```python
from build123d import *

# Parameters (mm, degrees)
F1_DEPTH     = 10
F2_DEPTH     = 8
F3_R         = 3
F4_T1_DEPTH  = 21.25
F4_T4_ANGLE  = 90
F4_T6_ANGLE  = 90
F4_T8_ANGLE  = 90
F4_T10_ANGLE = 90
F4_T12_ANGLE = 90
F4_T14_ANGLE = 90
F4_T16_ANGLE = 90
F4_T18_ANGLE = 90


# Not quite as in the source:
# - a fillet or chamfer that OpenCascade refuses, or shapes differently, is made with other operations: its cross-section is extruded or revolved along the edge and cut away or added


with BuildPart() as f1:
    # F0 (on Top) → F1 (new body)
    with BuildSketch(Plane.XY):
        Polygon((25.7107810123, -8.5209181738), (27.2851523571, -8.9427697042), (27.7070038876, -10.5171410491), (33.0728534806, -15.8829906421), (49.6898628385, 0.7340187158), (36.9619407771, 13.4619407771), (20.3449314192, -3.1550685808), align=None)
        Polygon((33.0728534806, -15.8829906421), (27.7070038876, -10.5171410491), (29.8254495283, -18.4232878133), (22.8852285904, -25.3635087511), (14.9790818262, -23.2450631104), (20.3449314192, -28.6109127035), align=None)
        Polygon((17.8046342481, -6.4024725331), (25.7107810123, -8.5209181738), (20.3449314192, -3.1550685808), (7.6170093579, -15.8829906421), (12.9828589509, -21.2488402351), (10.8644133102, -13.342693471), align=None)
        Polygon((49.6898628385, -32.5), (33.0728534806, -15.8829906421), (20.3449314192, -28.6109127035), (36.9619407771, -45.2279220614), align=None)
        Polygon((7.6170093579, -15.8829906421), (20.3449314192, -3.1550685808), (3.7279220614, 13.4619407771), (-9, 0.7340187158), align=None)
        Polygon((3.7279220614, -45.2279220614), (20.3449314192, -28.6109127035), (14.9790818262, -23.2450631104), (13.4047104814, -22.82321158), (12.9828589509, -21.2488402351), (7.6170093579, -15.8829906421), (-9, -32.5), align=None)
        Polygon((29.8254495283, -18.4232878133), (27.7070038876, -10.5171410491), (25.7107810123, -8.5209181738), (17.8046342481, -6.4024725331), (10.8644133102, -13.342693471), (12.9828589509, -21.2488402351), (14.9790818262, -23.2450631104), (22.8852285904, -25.3635087511), align=None)
        Polygon((27.7070038876, -10.5171410491), (27.2851523571, -8.9427697042), (25.7107810123, -8.5209181738), align=None)
        Polygon((13.4047104814, -22.82321158), (14.9790818262, -23.2450631104), (12.9828589509, -21.2488402351), align=None)
    extrude(amount=F1_DEPTH)

    # F0 (on Top) → F2 (cut)
    with BuildSketch(Plane.XY):
        Polygon((29.8254495283, -18.4232878133), (27.7070038876, -10.5171410491), (25.7107810123, -8.5209181738), (17.8046342481, -6.4024725331), (10.8644133102, -13.342693471), (12.9828589509, -21.2488402351), (14.9790818262, -23.2450631104), (22.8852285904, -25.3635087511), align=None)
        Polygon((13.4047104814, -22.82321158), (14.9790818262, -23.2450631104), (12.9828589509, -21.2488402351), align=None)
        Polygon((27.7070038876, -10.5171410491), (27.2851523571, -8.9427697042), (25.7107810123, -8.5209181738), align=None)
    extrude(amount=F2_DEPTH, mode=Mode.SUBTRACT)

    # F3
    f3_edges = [f1.edges().sort_by_distance(p)[0] for p in [
        (43.325902, 7.09798, 10),
        (28.653436, 5.153436, 10),
        (12.036427, 5.153436, 10),
        (-2.636039, 7.09798, 10),
        (-0.691495, -7.574486, 10),
        (-0.691495, -24.191495, 10),
        (-2.636039, -38.863961, 10),
        (12.036427, -36.919417, 10),
        (28.653436, -36.919417, 10),
        (43.325902, -38.863961, 10),
        (41.381358, -24.191495, 10),
        (41.381358, -7.574486, 10),
    ]]
    fillet(f3_edges, radius=F3_R)

    # F4: fillet of radius 4.5 on 8 edges, made by hand

    # F4_s2 → F4_t1 (cut)
    with BuildSketch(Plane.XY.offset(-11.25)):
        with BuildLine():
            ThreePointArc((40.1439212925, 10.2799602618), (36.9619407771, 11.5979797464), (33.7799602618, 10.2799602618))
            Line((33.7799602618, 10.2799602618), (36.9619407771, 13.4619407771))
            Line((36.9619407771, 13.4619407771), (40.1439212925, 10.2799602618))
        make_face()
        with BuildLine():
            ThreePointArc((46.5078823231, 3.9159992311), (47.8259018078, 0.7340187158), (46.5078823231, -2.4479617996))
            Line((46.5078823231, -2.4479617996), (49.6898628385, 0.7340187158))
            Line((49.6898628385, 0.7340187158), (46.5078823231, 3.9159992311))
        make_face()
        with BuildLine():
            ThreePointArc((46.5078823231, -29.3180194847), (47.8259018078, -32.5), (46.5078823231, -35.6819805153))
            Line((46.5078823231, -35.6819805153), (49.6898628385, -32.5))
            Line((49.6898628385, -32.5), (46.5078823231, -29.3180194847))
        make_face()
        with BuildLine():
            ThreePointArc((40.1439212925, -42.045941546), (36.9619407771, -43.3639610307), (33.7799602618, -42.045941546))
            Line((33.7799602618, -42.045941546), (36.9619407771, -45.2279220614))
            Line((36.9619407771, -45.2279220614), (40.1439212925, -42.045941546))
        make_face()
        with BuildLine():
            ThreePointArc((6.9099025767, -42.045941546), (3.7279220614, -43.3639610307), (0.545941546, -42.045941546))
            Line((0.545941546, -42.045941546), (3.7279220614, -45.2279220614))
            Line((3.7279220614, -45.2279220614), (6.9099025767, -42.045941546))
        make_face()
        with BuildLine():
            ThreePointArc((-5.8180194847, -29.3180194847), (-7.1360389693, -32.5), (-5.8180194847, -35.6819805153))
            Line((-5.8180194847, -35.6819805153), (-9, -32.5))
            Line((-9, -32.5), (-5.8180194847, -29.3180194847))
        make_face()
        with BuildLine():
            ThreePointArc((-5.8180194847, 3.9159992311), (-7.1360389693, 0.7340187158), (-5.8180194847, -2.4479617996))
            Line((-5.8180194847, -2.4479617996), (-9, 0.7340187158))
            Line((-9, 0.7340187158), (-5.8180194847, 3.9159992311))
        make_face()
        with BuildLine():
            ThreePointArc((6.9099025767, 10.2799602618), (3.7279220614, 11.5979797464), (0.545941546, 10.2799602618))
            Line((0.545941546, 10.2799602618), (3.7279220614, 13.4619407771))
            Line((3.7279220614, 13.4619407771), (6.9099025767, 10.2799602618))
        make_face()
    extrude(amount=F4_T1_DEPTH, mode=Mode.SUBTRACT)

    # F4_s3 → F4_t4 (revolve, cut)
    with BuildSketch(Plane(origin=(-1.6850288425, 1.6850288425, 0), x_dir=(0, 0, 1), z_dir=(0.7071067812, -0.7071067812, 0))):
        with BuildLine():
            ThreePointArc((10, -9.1550685808), (9.1213203436, -11.2763889243), (7, -12.1550685808))
            Line((7, -12.1550685808), (10, -12.1550685808))
            Line((10, -12.1550685808), (10, -9.1550685808))
        make_face()
    revolve(axis=Axis((3.7279220614, 7.0979797464, 10), (0, 0, 1)), revolution_arc=F4_T4_ANGLE, mode=Mode.SUBTRACT)

    # F4_s5 → F4_t6 (revolve, cut)
    with BuildSketch(Plane(origin=(-0.9510101268, -0.9510101268, 0), x_dir=(0, 0, 1), z_dir=(0.7071067812, 0.7071067812, 0))):
        with BuildLine():
            ThreePointArc((10, -3.8829906421), (9.1213203436, -6.0043109857), (7, -6.8829906421))
            Line((7, -6.8829906421), (10, -6.8829906421))
            Line((10, -6.8829906421), (10, -3.8829906421))
        make_face()
    revolve(axis=Axis((-2.6360389693, 0.7340187158, 10), (0, 0, 1)), revolution_arc=F4_T6_ANGLE, mode=Mode.SUBTRACT)

    # F4_s7 → F4_t8 (revolve, cut)
    with BuildSketch(Plane(origin=(-17.5680194847, -17.5680194847, 0), x_dir=(0, 0, 1), z_dir=(0.7071067812, 0.7071067812, 0))):
        with BuildLine():
            ThreePointArc((10, 19.6170093579), (9.1213203436, 17.4956890143), (7, 16.6170093579))
            Line((7, 16.6170093579), (10, 16.6170093579))
            Line((10, 16.6170093579), (10, 19.6170093579))
        make_face()
    revolve(axis=Axis((-2.6360389693, -32.5, 10), (0, 0, 1)), revolution_arc=F4_T8_ANGLE, mode=Mode.SUBTRACT)

    # F4_s9 → F4_t10 (revolve, cut)
    with BuildSketch(Plane(origin=(21.295941546, -21.295941546, 0), x_dir=(0, 0, 1), z_dir=(-0.7071067812, 0.7071067812, 0))):
        with BuildLine():
            ThreePointArc((10, -26.3449314192), (9.1213203436, -28.4662517628), (7, -29.3449314192))
            Line((7, -29.3449314192), (10, -29.3449314192))
            Line((10, -29.3449314192), (10, -26.3449314192))
        make_face()
    revolve(axis=Axis((3.7279220614, -38.8639610307, 10), (0, 0, 1)), revolution_arc=F4_T10_ANGLE, mode=Mode.SUBTRACT)

    # F4_s11 → F4_t12 (revolve, cut)
    with BuildSketch(Plane(origin=(37.9129509039, -37.9129509039, 0), x_dir=(0, 0, 1), z_dir=(-0.7071067812, 0.7071067812, 0))):
        with BuildLine():
            ThreePointArc((10, -2.8449314192), (9.1213203436, -4.9662517628), (7, -5.8449314192))
            Line((7, -5.8449314192), (10, -5.8449314192))
            Line((10, -5.8449314192), (10, -2.8449314192))
        make_face()
    revolve(axis=Axis((36.9619407771, -38.8639610307, 10), (0, 0, 1)), revolution_arc=F4_T12_ANGLE, mode=Mode.SUBTRACT)

    # F4_s13 → F4_t14 (revolve, cut)
    with BuildSketch(Plane(origin=(5.4129509039, 5.4129509039, 0), x_dir=(0, 0, 1), z_dir=(-0.7071067812, -0.7071067812, 0))):
        with BuildLine():
            ThreePointArc((10, -55.1170093579), (9.1213203436, -57.2383297014), (7, -58.1170093579))
            Line((7, -58.1170093579), (10, -58.1170093579))
            Line((10, -58.1170093579), (10, -55.1170093579))
        make_face()
    revolve(axis=Axis((43.3259018078, -32.5, 10), (0, 0, 1)), revolution_arc=F4_T14_ANGLE, mode=Mode.SUBTRACT)

    # F4_s15 → F4_t16 (revolve, cut)
    with BuildSketch(Plane(origin=(22.0299602618, 22.0299602618, 0), x_dir=(0, 0, 1), z_dir=(-0.7071067812, -0.7071067812, 0))):
        with BuildLine():
            ThreePointArc((10, -31.6170093579), (9.1213203436, -33.7383297014), (7, -34.6170093579))
            Line((7, -34.6170093579), (10, -34.6170093579))
            Line((10, -34.6170093579), (10, -31.6170093579))
        make_face()
    revolve(axis=Axis((43.3259018078, 0.7340187158, 10), (0, 0, 1)), revolution_arc=F4_T16_ANGLE, mode=Mode.SUBTRACT)

    # F4_s17 → F4_t18 (revolve, cut)
    with BuildSketch(Plane(origin=(14.9319805153, -14.9319805153, 0), x_dir=(0, 0, 1), z_dir=(0.7071067812, -0.7071067812, 0))):
        with BuildLine():
            ThreePointArc((10, -32.6550685808), (9.1213203436, -34.7763889243), (7, -35.6550685808))
            Line((7, -35.6550685808), (10, -35.6550685808))
            Line((10, -35.6550685808), (10, -32.6550685808))
        make_face()
    revolve(axis=Axis((36.9619407771, 7.0979797464, 10), (0, 0, 1)), revolution_arc=F4_T18_ANGLE, mode=Mode.SUBTRACT)


solid = f1.part
```
Model file for the job. Use its own axes, mm. A direction names the side the tool comes from. Round coordinates to 2 decimals unless told otherwise and drop trailing zeros. Loops run counter-clockwise (first coordinate to the right, second up) from the corner with the lowest first, then second, coordinate; pieces in that order, holes last. Notation, with made-up numbers: M 32,15.5 L 88,15.5 A31 ccw 88,52.5 Z; hole C 28,-11.5 d1. An arc over 180 degrees is marked long. Put each result on its own line as item: value. Start each with the question number.
Item 1: Drop flat-ended pins along their axis: P1, Ø4, axis at y = -20, z = 7.5, coming from the +X side; P2, Ø5.5, axis at x = 18.5, y = -11, coming from the -Z side. Give the stop position or say it passes through.
Item 2: Drill centre lines: line 1 along Z through (x, y) = (17, -22); line 2 along Y through (x, z) = (43, 7.25); line 3 along X through (y, z) = (-17, 7.75). Where is each one in solid material? Low to high.
Item 3: 3-axis set-ups, long thin cutter, end or side, ignore diameter. For faces 1 (the face through (-2.043, 6.416, 9.145)), 2 (the face through (13.72, 3.47, 3.45)), 3 (the face through (26.31, -21.94, 3.94)), 4 (the face through (1, -22.5, 3.5)), 5 (the face through (13.533, -35.422, 3.451)): which of +Z, -Z, +X, -X, +Y, -Y reach the whole face in a straight line?
Item 4: Mould opens along X. For faces 6 (the face through (-1.954, -38.271, 9.145)), 7 (the face through (42.643, 6.505, 9.145)), 8 (the face through (27.2, 3.7, 3.5)) say: released by +X, released by -X, zero draft, split by the parting line, or undercut.
Item 5: Cut at A-A (z = 0.75). List the corners of the cut face in (x, y).
Answer block:
1. P1: x = 39.16
1. P2: z = 8
2. line 1: 8 to 10
2. line 2: -39.18 to -25.82, -5.94 to 7.41
2. line 3: 6.63 to 11.84, 29.44 to 34.06
3. face 1: +Z, -X, +Y
3. face 2: +Z, -Z, +Y
3. face 3: -Z
3. face 4: +Z, -Z, -X
3. face 5: +Z, -Z, -Y
4. face 6: released by -X
4. face 7: released by +X
4. face 8: undercut
5. outline: M -5.82,-35.68 L 0.55,-42.05 A4.5 ccw 6.91,-42.05 L 20.34,-28.61 L 33.78,-42.05 A4.5 ccw 40.14,-42.05 L 46.51,-35.68 A4.5 ccw 46.51,-29.32 L 33.07,-15.88 L 46.51,-2.45 A4.5 ccw 46.51,3.92 L 40.14,10.28 A4.5 ccw 33.78,10.28 L 20.34,-3.16 L 6.91,10.28 A4.5 ccw 0.55,10.28 L -5.82,3.92 A4.5 ccw -5.82,-2.45 L 7.62,-15.88 L -5.82,-29.32 A4.5 ccw Z; hole M 10.86,-13.34 L 13.4,-22.82 L 22.89,-25.36 L 29.83,-18.42 L 27.29,-8.94 L 17.8,-6.4 Z
